Part model, mm, in its own coordinate system. Face numbers are marked on the shaded views. A direction names the side the tool comes from. Round coordinates to 2 decimals unless told otherwise and drop trailing zeros. Order: outer loops, then holes, each group sorted by start corner. A loop starts at its lowest first (then second) coordinate and runs counter-clockwise, first axis right, second up. Notation, with made-up numbers: (83.25, 86) - (107.25, 86) arc R15 ccw to (107.25, 108) - close; hole circle Ø1 at (61.5, -38). An arc over 180 degrees is marked (long way). Answer as a JSON object with one key per item and string values.
```python
from build123d import *

# Parameters (mm, degrees)
EXTRUDE_1_DEPTH      = 50
EXTRUDE_START        = -4
EXTRUDE_2_DEPTH      = 46
CUT_EXTRUDE_1_DEPTH  = 92.1
CUT_EXTRUDE_START    = 94.5
CUT_EXTRUDE_2_DEPTH  = 241.890744243
SKETCH_17_W          = 5
SKETCH_17_H          = 88.9
SKETCH_17_H_2        = 46.554557274
SKETCH_17_H_3        = 30
SKETCH_17_H_4        = 15
SKETCH_17_H_5        = 12
CUT_EXTRUDE_5_DEPTH  = 30
SKETCH_37_R          = 1.9
CUT_EXTRUDE_13_DEPTH = 174.81246936


with BuildPart() as part:
    # 草图1 → 凸台-拉伸1 (new body)
    with BuildSketch(Plane.XY):
        with BuildLine():
            Line((-22.183039724, 96.9), (-73.14723658, 33.490663373))
            ThreePointArc((-73.14723658, 33.490663373), (-73.966258204, 32.018718559), (-74.25, 30.358324465))
            Line((-74.25, 30.358324465), (-74.25, 5))
            ThreePointArc((-74.25, 5), (-72.785533906, 1.464466094), (-69.25, 0))
            Line((-69.25, 0), (69.25, 0))
            ThreePointArc((69.25, 0), (72.785533906, 1.464466094), (74.25, 5))
            Line((74.25, 5), (74.25, 30.358324465))
            ThreePointArc((74.25, 30.358324465), (73.966258204, 32.018718559), (73.14723658, 33.490663373))
            Line((73.14723658, 33.490663373), (22.183039724, 96.9))
            Line((22.183039724, 96.9), (-22.183039724, 96.9))
        make_face()
        with BuildLine():
            ThreePointArc((-69.25, 2.4), (-71.088477631, 3.161522369), (-71.85, 5))
            Line((-71.85, 5), (-71.85, 30.358324465))
            ThreePointArc((-71.85, 30.358324465), (-71.702454266, 31.221729394), (-71.276563022, 31.987140697))
            Line((-71.276563022, 31.987140697), (-21.032894864, 94.5))
            Line((-21.032894864, 94.5), (21.032894864, 94.5))
            Line((21.032894864, 94.5), (71.276563022, 31.987140697))
            ThreePointArc((71.276563022, 31.987140697), (71.702454266, 31.221729394), (71.85, 30.358324465))
            Line((71.85, 30.358324465), (71.85, 5))
            ThreePointArc((71.85, 5), (71.088477631, 3.161522369), (69.25, 2.4))
            Line((69.25, 2.4), (-69.25, 2.4))
        make_face(mode=Mode.SUBTRACT)
    extrude(amount=EXTRUDE_1_DEPTH)

    # 草图2 → Extrude 2 (add)
    with BuildSketch(Plane(origin=(0, 0, 0), x_dir=(-1, 0, 0), z_dir=(0, 0, -1)).offset(EXTRUDE_START)):
        with BuildLine():
            Line((-100, 96.9), (-100, 0))
            Line((-100, 0), (-69.25, 0))
            ThreePointArc((-69.25, 0), (-72.785533906, 1.464466094), (-74.25, 5))
            Line((-74.25, 5), (-74.25, 30.358324465))
            ThreePointArc((-74.25, 30.358324465), (-73.966258204, 32.018718559), (-73.14723658, 33.490663373))
            Line((-73.14723658, 33.490663373), (-22.183039724, 96.9))
            Line((-22.183039724, 96.9), (-100, 96.9))
        make_face()
    extrude_2 = extrude(amount=-EXTRUDE_2_DEPTH)

    # 草图4 → Cut-Extrude 1 (cut)
    with BuildSketch(Plane.XZ.offset(-94.5)):
        Polygon((21.032894864, 50), (21.032894864, 8.470679814), (97.6, 24.745520419), (97.6, 50), align=None)
    cut_extrude_1 = extrude(amount=CUT_EXTRUDE_1_DEPTH, mode=Mode.SUBTRACT)

    # 草图4<4> → 切除-拉伸2 (cut, through all)
    with BuildSketch(Plane.XZ.offset(-94.5).offset(CUT_EXTRUDE_START)):
        Polygon((97.6, 4), (97.6, 20.470256304), (74.25, 4), align=None)
        Polygon((100, 22.163130613), (97.6, 20.470256304), (97.6, 4), (100, 4), align=None)
    cut_extrude_2 = extrude(amount=-CUT_EXTRUDE_2_DEPTH, mode=Mode.SUBTRACT)

    # 镜向1: Extrude 2, Cut-Extrude 1, 切除-拉伸2 across plane
    add(extrude_2.mirror(Plane(origin=(0, 0, 0), x_dir=(0, 0, 1), z_dir=(1, 0, 0))))
    add(cut_extrude_1.mirror(Plane(origin=(0, 0, 0), x_dir=(0, 0, 1), z_dir=(1, 0, 0))), mode=Mode.SUBTRACT)
    add(cut_extrude_2.mirror(Plane(origin=(0, 0, 0), x_dir=(0, 0, 1), z_dir=(1, 0, 0))), mode=Mode.SUBTRACT)

    # 草图17 → Cut-Extrude 5 (cut)
    with BuildSketch(Plane(origin=(0, 0, 4), x_dir=(-1, 0, 0), z_dir=(0, 0, -1))):
        with Locations((-90, 48.45)):
            Rectangle(SKETCH_17_W, SKETCH_17_H)
        with Locations((-80, 48.45)):
            Rectangle(SKETCH_17_W, SKETCH_17_H)
        with Locations((-70, 69.622721363)):
            Rectangle(SKETCH_17_W, SKETCH_17_H_2)
        with Locations((-60, 77.9)):
            Rectangle(SKETCH_17_W, SKETCH_17_H_3)
        with Locations((-50, 85.4)):
            Rectangle(SKETCH_17_W, SKETCH_17_H_4)
        with Locations((-40, 86.9)):
            Rectangle(SKETCH_17_W, SKETCH_17_H_5)
    cut_extrude_5 = extrude(amount=-CUT_EXTRUDE_5_DEPTH, mode=Mode.SUBTRACT)

    # 镜向2: Cut-Extrude 5 across plane
    add(cut_extrude_5.mirror(Plane(origin=(0, 0, 0), x_dir=(0, 0, 1), z_dir=(1, 0, 0))), mode=Mode.SUBTRACT)

    # 草图37 → 切除-拉伸13 (cut, through all)
    with BuildSketch(Plane(origin=(-58.922506005, 47.35798157, 0), x_dir=(0, 0, -1), z_dir=(0.7794473160570582, -0.6264677816866949, 0))):
        with Locations(Location((-6.5, 56.48134038, 0), (0, 0, 90))):
            Circle(SKETCH_37_R)
    cut_extrude_13 = extrude(amount=-CUT_EXTRUDE_13_DEPTH, mode=Mode.SUBTRACT)

    # 镜向4: 切除-拉伸13 across plane
    add(cut_extrude_13.mirror(Plane(origin=(0, 0, 0), x_dir=(0, 0, 1), z_dir=(1, 0, 0))), mode=Mode.SUBTRACT)


solid = part.part
```
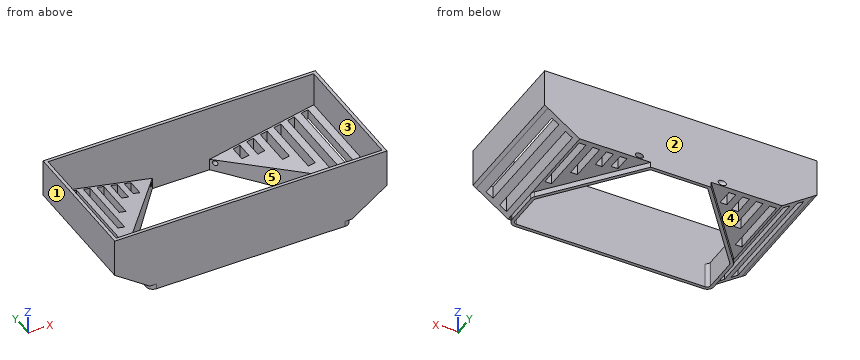
Item 1: Cut at A-A (y = 22). State how many separate pieces and enclosed holes the cut face has, plus the area to 3 significant figures.
Taken from the geometry:
{"separate pieces": "6", "enclosed holes": "0", "area": "490 mm2"}
Item 2: Cut at C-C (x = -17.5). Write the cut outline in (y, z), plus the area to 3 significant figures.
Taken from the geometry:
{"outline": "(0, 0) - (2.4, 0) - (2.4, 50) - (0, 50) - close; (94.5, 0) - (96.9, 0) - (96.9, 50) - (94.5, 50) - close", "area": "240 mm2"}
Item 3: Tool access for the marked faces 1, 2, 3, 4 and 5: list every direction of +Z, -Z, +X, -X, +Y, -Y with a clear straight run to the whole face (end or side of a thin tool).
Taken from the geometry:
{"face 1": "+Z, -Z, -X, +Y, -Y", "face 2": "+Z, -Z, +X, -X, +Y", "face 3": "+Z", "face 4": "-Z, -X, +Y", "face 5": "+Z, -Z"}
Item 4: Drop flat-ended pins along their axis: P1, Ø1.5, axis at y = 74.5, z = 15.5, coming from the -X side; P2, Ø7, axis at y = 62, z = 8.5, coming from the -X side; P3, Ø7.5, axis at y = 68.5, z = 16, coming from the -X side. Give the stop position or say it passes through.
Taken from the geometry:
{"P1": "x = -87.5", "P2": "x = -85.59", "P3": "x = -96.58"}
Item 5: Probe L1, parallel to X at y = 19, z = 40.5; L2, parallel to Y at x = 20, z = 33; L3, parallel to Y at x = -40, z = 3. List the from-to ranges inside material, lowest first. Write a range as from..to.
Taken from the geometry:
{"L1": "-100..-97.6, 97.6..100", "L2": "0..2.4, 94.5..96.9", "L3": "0..2.4, 70.9..74.73"}
Item 6: Cut at B-B (z = 35). Write the cut outline in (x, y).
Taken from the geometry:
{"outline": "(-100, 0) - (100, 0) - (100, 96.9) - (-100, 96.9) - close; hole (-97.6, 2.4) - (97.6, 2.4) - (97.6, 94.5) - (-97.6, 94.5) - close"}
Item 7: Cut at D-D (x = 55.5). Write the cut outline in (y, z), plus the area to 3 significant figures.
Taken from the geometry:
{"outline": "(0, 0) - (2.4, 0) - (2.4, 50) - (0, 50) - close; (51.62, 0) - (55.45, 0) - (55.45, 4) - (96.9, 4) - (96.9, 50) - (94.5, 50) - (94.5, 15.8) - (51.62, 15.8) - close", "area": "752 mm2"}
